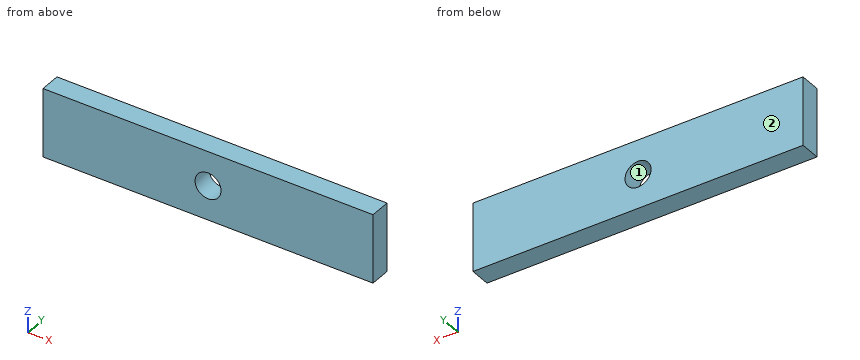
from build123d import *

# Parameters (mm, degrees)
SKETCH1_W              = 152.4
SKETCH1_H              = 31.75
BOSS_EXTRUDE1_DEPTH    = 4.7625
F_12_0MM_DOWEL_HOLE1_D = 12


with BuildPart() as part:
    # Sketch1 → Boss-Extrude1 (new, symmetric)
    with BuildSketch(Plane(origin=(0, 0, 0), x_dir=(1, 0, 0), z_dir=(0, 1, 0))):
        Rectangle(SKETCH1_W, SKETCH1_H)
    extrude(amount=BOSS_EXTRUDE1_DEPTH, both=True)

    # Ø12.0mm Dowel Hole1 (through all)
    with Locations(Plane(origin=(0, -4.7625, 0), x_dir=(-1, 0, 0), z_dir=(0, -1, 0))):
        with Locations((0, 0)):
            Hole(F_12_0MM_DOWEL_HOLE1_D / 2)


solid = part.part
Can you work these out from the model? Positions are in its coordinate system, mm. Face numbers are marked on the shaded views. Round coordinates to 2 decimals unless told otherwise and drop trailing zeros. Write each loop counter-clockwise with the first axis right and the second up, starting at its lowest first coordinate (ties: lowest second). Pieces come first, ordered by that corner, then holes. Notation, with made-up numbers: M -22.75,-26.5 L 17.25,-26.5 A15 ccw 17.25,-0.5 Z; hole C 46,75.5 d1. An arc over 180 degrees is marked long. Use a Markdown table: item, result.
Item 1: I want a section at A-A (z = 0). List the corners of the cut face in (x, y) for me.
Found:
| item | result |
|---|---|
| outline | M -76.2,-4.76 L -6,-4.76 L -6,4.76 L -76.2,4.76 Z; M 6,-4.76 L 76.2,-4.76 L 76.2,4.76 L 6,4.76 Z |
Item 2: We'd pull the mould along Z, two halves only. Please class the marked faces 1 and 2: released by +Z, released by -Z, zero draft, split by the parting line, or undercut.
Found:
| item | result |
|---|---|
| face 1 | undercut |
| face 2 | zero draft |
Item 3: If I drill on line 1 along Z through (x, y) = (0, 1.5) (3 decimals); line 2 along Z through (x, y) = (1.5, 2.25) (3 decimals); line 3 along X through (y, z) = (1.25, 1.5), over which ranges is the centre line in solid material (lowest first)? Write a range as [from, to].
Found:
| item | result |
|---|---|
| line 1 | z = [-15.875, -6], [6, 15.875] |
| line 2 | z = [-15.875, -5.809], [5.809, 15.875] |
| line 3 | x = [-76.2, -5.81], [5.81, 76.2] |
Item 4: I want a section at C-C (y = -1). List the corners of the cut face in (x, z) for me (3 decimals), and give its area (3 significant figures).
Found:
| item | result |
|---|---|
| outline | M -76.2,-15.875 L 76.2,-15.875 L 76.2,15.875 L -76.2,15.875 Z; hole C 0,0 d12 |
| area | 4,730 mm2 |
Item 5: I want a section at B-B (x = 0). List the corners of the cut face in (y, z) for me (1 decimal).
Found:
| item | result |
|---|---|
| outline | M -4.8,-15.9 L 4.8,-15.9 L 4.8,-6 L -4.8,-6 Z; M -4.8,6 L 4.8,6 L 4.8,15.9 L -4.8,15.9 Z |
